```python
from build123d import *

# Parameters (mm, degrees)
SKETCH2_W           = 1
SKETCH2_H           = 2
BOSS_EXTRUDE1_DEPTH = 8.5
FILLET1_R           = 1.5


with BuildPart() as part:
    # Sketch2 → Boss-Extrude1 (new body)
    with BuildSketch(Plane.XY):
        Polygon((-2.95, 55.75), (-7.75, 55.75), (-7.75, 45.75), (-2.95, 45.75), (-2.95, 47.75), align=None)
        Polygon((-7.75, 55.75), (-12.55, 55.75), (-12.55, 47.75), (-12.55, 45.75), (-7.75, 45.75), align=None)
        with Locations((-2.45, 46.75)):
            Rectangle(SKETCH2_W, SKETCH2_H)
        with Locations((-13.05, 46.75)):
            Rectangle(SKETCH2_W, SKETCH2_H)
    extrude(amount=BOSS_EXTRUDE1_DEPTH)

    # Fillet1
    fillet1_edges = [part.edges().sort_by_distance(p)[0] for p in [
        (-2.95, 51.75, 0),
        (-12.55, 51.75, 8.5),
        (-12.55, 51.75, 0),
        (-7.75, 55.75, 0),
        (-2.95, 55.75, 4.25),
        (-12.55, 55.75, 4.25),
        (-2.95, 51.75, 8.5),
        (-7.75, 55.75, 8.5),
    ]]
    fillet(fillet1_edges, radius=FILLET1_R)


solid = part.part
```
Check sheet for the modelled part. Datum: model origin and axes. Units: mm. A direction names the side the tool comes from. Round coordinates to 2 decimals unless told otherwise and drop trailing zeros. Order: outer loops, then holes, each group sorted by start corner. A loop starts at its lowest first (then second) coordinate and runs counter-clockwise, first axis right, second up.
1) Section check D-D (y = 54.5). Record the boundary of the cut face in (x, z), and give its area (3 significant figures).
2) Tool access check on faces 1 (the cylindrical face through (-3.38, 51.05, 8.05)), 2 (the cylindrical face through (-12.12, 50.95, 0.45)), 3 (the flat face through (-2.95, 51, 4)), 4 (the cylindrical face through (-3.38, 51.05, 0.45)), 5 (the cylindrical face through (-12.12, 50.95, 8.05)). Record the directions out of +Z, -Z, +X, -X, +Y, -Y that give a thin tool (end or side, any length) a straight path to the whole face; none if there is none.
3) Section check C-C (x = -4). Record the boundary of the cut face in (y, z), and give its area (3 significant figures).
4) Go/stop test with flat-tipped pins: pin 1 Ø0.8 at (x, z) = (-12.5, 2.5) entering from +Y; pin 2 Ø1 at (y, z) = (50, 3.5) entering from -X; pin 3 Ø1.6 at (y, z) = (51.5, 4.5) entering from +X. Record where each tip stops, or that it passes through.
5) Scan lines: line 1 (X direction, y = 48.75, z = 3.25); line 2 (Y direction, x = -3, z = 0.5). Record each from-to range of solid material in increasing order.
6) Section check A-A (z = 2.25). Record the boundary of the cut face in (x, y).
7) Section check B-B (y = 51.25). Record the boundary of the cut face in (x, z), and give its area (3 significant figures).
Result:
1. outline: (-12.53, 1.5) arc R1.48 ccw to (-11.05, 0.02) - (-4.45, 0.02) arc R1.48 ccw to (-2.97, 1.5) - (-2.97, 7) arc R1.48 ccw to (-4.45, 8.48) - (-11.05, 8.48) arc R1.48 ccw to (-12.53, 7) - close
1. area: 79.0 mm2
2. face 1: +Z, +X, +Y
2. face 2: -Z, -X, +Y
2. face 3: +Z, -Z, +X, +Y
2. face 4: -Z, +X, +Y
2. face 5: +Z, -X, +Y
3. outline: (45.75, 0) - (47.75, 0) - (47.75, 0.07) - (54.25, 0.07) arc R1.43 ccw to (55.68, 1.5) - (55.68, 7) arc R1.43 ccw to (54.25, 8.43) - (47.75, 8.43) - (47.75, 8.5) - (45.75, 8.5) - close
3. area: 82.4 mm2
4. pin 1: stops at y = 55.32
4. pin 2: stops at x = -12.55
4. pin 3: stops at x = -2.95
5. line 1: x = -12.55 to -2.95
5. line 2: y = 45.75 to 47.75
6. outline: (-13.55, 45.75) - (-1.95, 45.75) - (-1.95, 47.75) - (-2.95, 47.75) - (-2.95, 54.25) arc R1.5 ccw to (-4.45, 55.75) - (-11.05, 55.75) arc R1.5 ccw to (-12.55, 54.25) - (-12.55, 47.75) - (-13.55, 47.75) - close
7. outline: (-12.55, 1.5) arc R1.5 ccw to (-11.05, 0) - (-4.45, 0) arc R1.5 ccw to (-2.95, 1.5) - (-2.95, 7) arc R1.5 ccw to (-4.45, 8.5) - (-11.05, 8.5) arc R1.5 ccw to (-12.55, 7) - close
7. area: 79.7 mm2
